Source: three-view drawing plus pictorial views. Frame: mm from the lowest corner of the part. A direction names the side the tool comes from. Coordinates: 2 decimals unless noted, no trailing zeros. Order: outer loops, then holes, each group sorted by start corner. A loop starts at its lowest first (then second) coordinate and runs counter-clockwise, first axis right, second up. Notation, with made-up numbers: M -33,67 L -9,67 A21 cw -9,94 Z; hole C 41.25,16 d9. An arc over 180 degrees is marked long. Use CSV: the item, a comma, the result in double quotes. Start each with the question number.
Q1. Ray query, probe 1 along X at (y, z) = (28, 26.5); probe 2 along Y at (x, z) = (47, 48); probe 3 along Z at (x, y) = (9, 16). Return the intervals inside material, ascending.
Q2. Access query for the marked faces 1 and 2. Directions: +Z, -Z, +X, -X, +Y, -Y. A direction counts if a zero-diameter tool reaches every point of the face in a straight line with its end or side. Return the directions, or none.
Q3. Section query A-A, the plane z = 42.5. Output: boundary loops of the cut face in (x, y).
Q4. Mould query, pull axis Y, two halves, no side actions, for the marked faces 3, 4 and 5. Classes: +Y half, -Y half, draft (parallel to the pull), parting line (faces both ways), or undercut.
Q5. Section query B-B, the plane y = 5.5. Output: boundary loops of the cut face in (x, z).
Q6. Section query C-C, the plane x = 49.5. Output: boundary loops of the cut face in (y, z), and give its area (3 significant figures).
Q7. First-contact query: P1, Ø8, axis at x = 14.5, y = 19, coming from the -Z side; P2, Ø2.5, axis at x = 59, z = 8, coming from the +Y side; P3, Ø6, axis at x = 26.5, z = 12.5, coming from the +Y side. Flat tips, straight axial feed; report the tip coordinate or a pass-through.
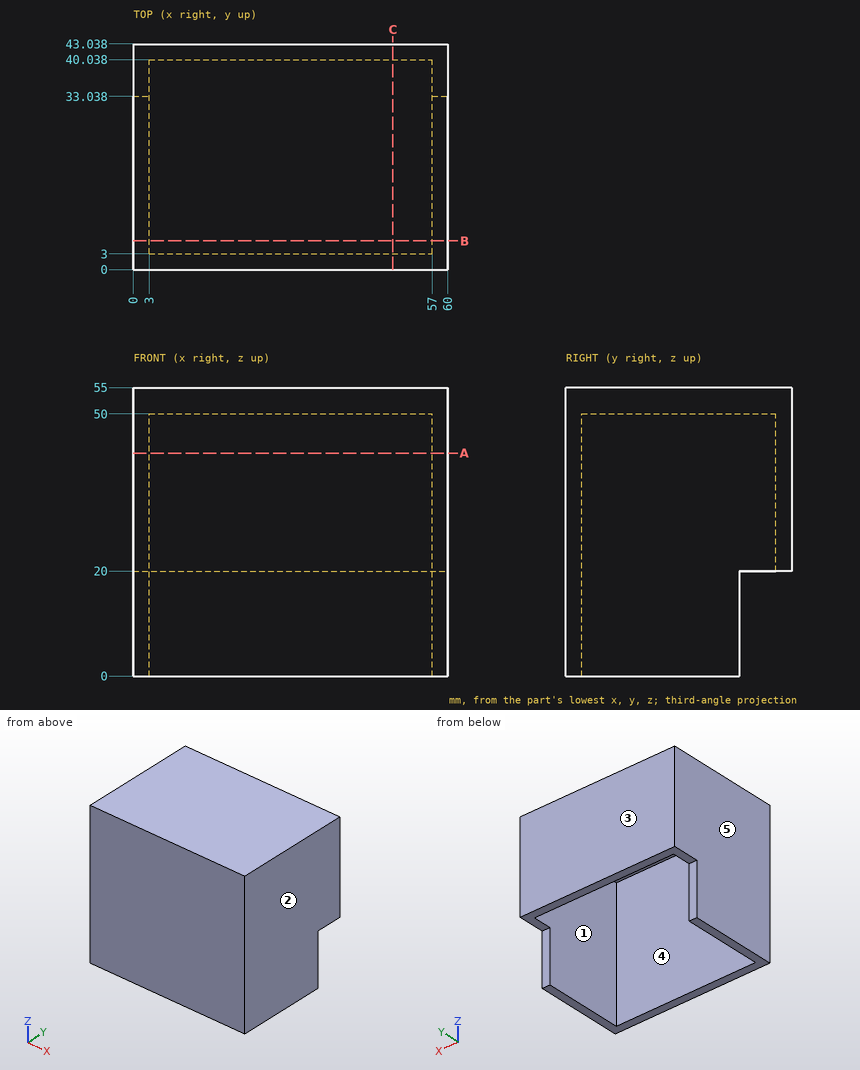
Responses:
1,probe 1,"x = 0 to 3, 57 to 60"
1,probe 2,"y = 0 to 3, 40.04 to 43.04"
1,probe 3,"z = 50 to 55"
2,face 1,"-Z"
2,face 2,"+Z, -Z, +X, +Y, -Y"
3,outline,"M 0,0 L 60,0 L 60,43.04 L 0,43.04 Z; hole M 3,3 L 57,3 L 57,40.04 L 3,40.04 Z"
4,face 3,"+Y half"
4,face 4,"undercut"
4,face 5,"draft"
5,outline,"M 0,0 L 3,0 L 3,50 L 57,50 L 57,0 L 60,0 L 60,55 L 0,55 Z"
6,outline,"M 0,0 L 3,0 L 3,50 L 40.04,50 L 40.04,20 L 43.04,20 L 43.04,55 L 0,55 Z"
6,area,"455 mm²"
7,P1,"stops at z = 50"
7,P2,"stops at y = 33.04"
7,P3,"stops at y = 3"
